Verification items for the finished model (mm, model axes). Face numbers are marked on the shaded views. A direction names the side the tool comes from. Coordinates: 2 decimals unless noted, no trailing zeros. Write each loop counter-clockwise with the first axis right and the second up, starting at its lowest first coordinate (ties: lowest second). Pieces come first, ordered by that corner, then holes. Notation, with made-up numbers: (4, -18.75) -> (51, -18.75) arc R27 cw to (51, 17.25) -> close; hole circle Ø2 at (66, -36.75). An arc over 180 degrees is marked (long way). Answer in a Markdown table with one row per item.
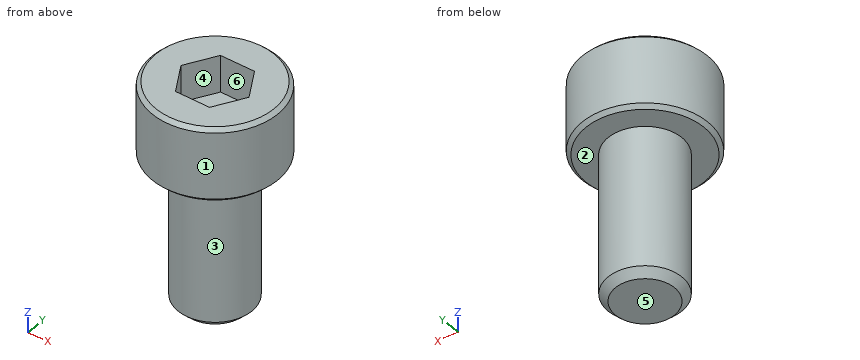
```python
from build123d import *

# Parameters (mm, degrees)
F3_DEPTH = 2.5
F4_SIZE  = 0.5
F5_SIZE  = 0.25


with BuildPart() as f1:
    # F0 (on Front) → F1 (revolve)
    with BuildSketch(Plane.XZ):
        Polygon((4.25, 0), (0, 0), (0, -15), (2.5, -15), (2.5, -5), (4.25, -5), align=None)
    revolve(axis=Axis((0, 0, -7.5), (0, 0, -1)))

    # F2 (on face) → F3 (cut)
    with BuildSketch(Plane.XY):
        Polygon((1.154701, 2), (-1.154701, 2), (-2.309401, 0), (-1.154701, -2), (1.154701, -2), (2.309401, 0), align=None)
    extrude(amount=-F3_DEPTH, mode=Mode.SUBTRACT)

    # F4
    f4_edges = [f1.edges().sort_by_distance(p)[0] for p in [
        (-2.5, 0, -15),
    ]]
    chamfer(f4_edges, length=F4_SIZE)

    # F5
    f5_edges = [f1.edges().sort_by_distance(p)[0] for p in [
        (-4.25, 0, 0),
        (-4.25, 0, -5),
    ]]
    chamfer(f5_edges, length=F5_SIZE)


solid = f1.part
```
1. Thickness scan on line 1 (X direction, y = 0, z = -13.75); line 2 (Y direction, x = -0.5, z = -0.75); line 3 (Y direction, x = 1.25, z = -0.75). Record the ranges inside material, lowest first. Write a range as from..to.
Geometry says:
| item | result |
|---|---|
| line 1 | -2.5..2.5 |
| line 2 | -4.22..-2, 2..4.22 |
| line 3 | -4.06..-1.83, 1.83..4.06 |
2. Depth check by flat-ended pin: P1, Ø1.5, axis at x = -1.5, z = -7.5, coming from the +Y side; P2, Ø1, axis at x = 1, y = -0.5, coming from the +Z side; P3, Ø1.5, axis at x = 2, z = -9.5, coming from the +Y side. Enter the tip coordinate at first touch or a pass-through.
Geometry says:
| item | result |
|---|---|
| P1 | y = 2.38 |
| P2 | z = -2.5 |
| P3 | y = 2.17 |
3. Section check B-B, the plane x = 0. Record the boundary of the cut face in (y, z), plus the area to 3 significant figures.
Geometry says:
| item | result |
|---|---|
| outline | (-4.25, -4.75) -> (-4, -5) -> (-2.5, -5) -> (-2.5, -14.5) -> (-2, -15) -> (2, -15) -> (2.5, -14.5) -> (2.5, -5) -> (4, -5) -> (4.25, -4.75) -> (4.25, -0.25) -> (4, 0) -> (2, 0) -> (2, -2.5) -> (-2, -2.5) -> (-2, 0) -> (-4, 0) -> (-4.25, -0.25) -> close |
| area | 82.1 mm^2 |
4. Section check A-A, the plane z = -1. Record the boundary of the cut face in (x, y), plus the area to 3 significant figures.
Geometry says:
| item | result |
|---|---|
| outline | circle Ø8.5 at (0, 0); hole (-2.31, 0) -> (-1.15, -2) -> (1.15, -2) -> (2.31, 0) -> (1.15, 2) -> (-1.15, 2) -> close |
| area | 42.9 mm^2 |
5. Mould release check, pull along Y, two halves, no side actions. Record for the marked faces 3, 4, 5 and 6: released by +Y, released by -Y, zero draft, split by the parting line, or undercut.
Geometry says:
| item | result |
|---|---|
| face 3 | split by the parting line |
| face 4 | undercut |
| face 5 | zero draft |
| face 6 | undercut |
6. Section check C-C, the plane z = -9.25. Record the boundary of the cut face in (x, y), plus the area to 3 significant figures.
Geometry says:
| item | result |
|---|---|
| outline | circle Ø5 at (0, 0) |
| area | 19.6 mm^2 |
7. Tool access check on the marked faces 1 and 2. Record the directions out of +Z, -Z, +X, -X, +Y, -Y that give a thin tool (end or side, any length) a straight path to the whole face; none if there is none.
Geometry says:
| item | result |
|---|---|
| face 1 | +Z, -Z |
| face 2 | -Z |
